```python
from build123d import *

# Parameters (mm, degrees)
SKETCH1_R           = 4.9999999999999964
BOSS_EXTRUDE1_DEPTH = 5
BOSS_EXTRUDE2_DEPTH = 70
BOSS_EXTRUDE3_DEPTH = 70
CUT_EXTRUDE1_DEPTH  = 5
SKETCH6_R           = 20.000000000000004
CUT_EXTRUDE2_DEPTH  = 1
CUT_EXTRUDE3_DEPTH  = 19.000000000000004
BOSS_EXTRUDE4_DEPTH = 1.9999999999999896
FILLET1_R           = 5


with BuildPart() as part:
    # Sketch1 → Boss-Extrude1 (new body)
    with BuildSketch(Plane.XY):
        with BuildLine():
            Line((-7.704615384615421, -40.00000000000001), (32.295384615384584, -40.00000000000001))
            ThreePointArc((32.295384615384584, -40.00000000000001), (72.29538461538459, 0), (32.29538461538458, 39.99999999999999))
            Line((32.29538461538458, 39.99999999999999), (-7.7046153846154315, 39.99999999999999))
            Line((-7.7046153846154315, 39.99999999999999), (-7.704615384615421, -40.00000000000001))
        make_face()
        with Locations((32.295384615384584, 0)):
            Circle(SKETCH1_R, mode=Mode.SUBTRACT)
    boss_extrude1 = extrude(amount=BOSS_EXTRUDE1_DEPTH)

    # Sketch2 → Boss-Extrude2 (add)
    with BuildSketch(Plane.XY.offset(5)):
        Polygon((-7.7046153846154315, 39.99999999999999), (-2.70461538461543, 39.99999999999999), (-2.7046153846154235, -40.00000000000001), (-7.704615384615421, -40.00000000000001), align=None)
    extrude(amount=BOSS_EXTRUDE2_DEPTH)

    # Mirror1: Boss-Extrude1 across plane
    add(boss_extrude1.mirror(Plane.XY.offset(40)))

    # Sketch4 → Boss-Extrude3 (add)
    with BuildSketch(Plane.XY.offset(5)):
        with BuildLine():
            Line((-2.7046153846154266, -40.00000000000001), (-2.7046153846154266, -30.000000000000007))
            Line((-2.7046153846154266, -30.000000000000007), (43.497251593214216, -30.000000000000007))
            Line((43.497251593214216, -30.000000000000007), (58.7528977260305, -30.000000000000007))
            ThreePointArc((58.7528977260305, -30.000000000000007), (46.43752023911554, -37.41657386773942), (32.295384615384584, -40.00000000000001))
            Line((32.295384615384584, -40.00000000000001), (-2.7046153846154266, -40.00000000000001))
        make_face()
    extrude(amount=BOSS_EXTRUDE3_DEPTH)

    # Sketch5 → Cut-Extrude1 (cut)
    with BuildSketch(Plane.ZY.offset(7.704615384615426)):
        with BuildLine():
            ThreePointArc((50.00000000000001, -1.388e-14), (43.82683432365097, 9.238795325112829), (32.92893218813463, 7.071067811865561))
            Line((32.92893218813452, 7.0710678118654755), (47.071067811865476, -7.071067811865483))
            ThreePointArc((47.0710678118656, -7.0710678118653725), (49.2387953251129, -3.826834323650836), (50.00000000000001, -1.633e-14))
        make_face()
        with BuildLine():
            Line((47.071067811865476, -7.071067811865483), (32.92893218813452, 7.0710678118654755))
            ThreePointArc((32.92893218813463, 7.071067811865561), (32.92893218813454, -7.071067811865502), (47.0710678118656, -7.0710678118653725))
        make_face()
    extrude(amount=-CUT_EXTRUDE1_DEPTH, mode=Mode.SUBTRACT)

    # Sketch6 → Cut-Extrude2 (cut)
    with BuildSketch(Plane.ZY.offset(7.704615384615426)):
        with Locations(Location((40.00000000000001, -1.388e-14, 0), (0, 0, 270))):
            Circle(SKETCH6_R)
    extrude(amount=-CUT_EXTRUDE2_DEPTH, mode=Mode.SUBTRACT)

    # Sketch7 → Cut-Extrude3 (cut)
    with BuildSketch(Plane(origin=(0, -30.000000000000007, 0), x_dir=(1, 0, 0), z_dir=(0, 1, 0))):
        Polygon((58.7528977260305, -53.00000000000001), (58.7528977260305, -40.00000000000001), (58.7528977260305, -27.000000000000004), (19.339689979409883, -27.000000000000007), (19.339689979409883, -53.00000000000001), align=None)
    extrude(amount=-CUT_EXTRUDE3_DEPTH, mode=Mode.SUBTRACT)

    # Sketch8 → Boss-Extrude4 (add)
    with BuildSketch(Plane(origin=(0, -30.000000000000007, 0), x_dir=(1, 0, 0), z_dir=(0, 1, 0))):
        Polygon((58.7528977260305, -53.00000000000001), (19.33968997940988, -53.00000000000001), (19.33968997940988, -27.000000000000007), (58.7528977260305, -27.000000000000004), (58.7528977260305, -25.000000000000007), (56.7528977260305, -25.000000000000007), (17.33968997940988, -25.000000000000007), (17.33968997940988, -55.00000000000001), (58.7528977260305, -55.00000000000001), align=None)
    extrude(amount=BOSS_EXTRUDE4_DEPTH)

    # Fillet1
    fillet1_edges = [part.edges().sort_by_distance(p)[0] for p in [
        (-7.704615384615421, -40.00000000000001, 40),
        (28.024141170707534, -30.000000000000007, 5),
        (28.024141170707537, -30.000000000000007, 75),
    ]]
    fillet(fillet1_edges, radius=FILLET1_R)


solid = part.part
```
For this review, take the finished solid that the model builds, in its own axes (mm). A direction names the side the tool comes from. Coordinates: 2 decimals unless noted, no trailing zeros. Order: outer loops, then holes, each group sorted by start corner. A loop starts at its lowest first (then second) coordinate and runs counter-clockwise, first axis right, second up. Notation, with made-up numbers: (-3.5, 69.25) -> (33.5, 69.25) arc R26 cw to (33.5, 83.25) -> close; hole circle Ø5 at (-14, -13.75). An arc over 180 degrees is marked (long way). Answer as CSV lines item,"result".
Q1. Clearance check with flat-ended pins moving along their axes: pin 1 Ø0.6 at (y, z) = (-29.5, 54) entering from +X; pin 2 Ø12 at (x, z) = (55.5, 64.5) entering from +Y; pin 3 Ø6 at (y, z) = (-36, 40) entering from +X; pin 4 Ø18 at (y, z) = (0, 40) entering from +X. State where each tip first meets the part, or that it passes through.
Model answer:
pin 1,"stops at x = 58.75"
pin 2,"stops at y = -29.97"
pin 3,"stops at x = 19.34"
pin 4,"passes through"
Q2. For faces 5 (the face through (34, -34, 27)), 6 (the face through (23, 1, 80)), 7 (the face through (34, 8, 75)), list the 3-axis set-ups (+Z, -Z, +X, -X, +Y, -Y) from which the entire face can be reached by the end or side of a thin tool; tool diameter is ignored.
Model answer:
face 5,"+X, +Y, -Y"
face 6,"+Z, +X, -X, +Y, -Y"
face 7,"+X, +Y"
Q3. We need section B-B (y = 0). State the section outline as (x, z) points, plus the area to 3 significant figures.
Model answer:
outline,"(-7.7, 0) -> (27.3, 0) -> (27.3, 5) -> (-2.7, 5) -> (-2.7, 30) -> (-6.7, 30) -> (-6.7, 20) -> (-7.7, 20) -> close; (-7.7, 60) -> (-6.7, 60) -> (-6.7, 50) -> (-2.7, 50) -> (-2.7, 75) -> (27.3, 75) -> (27.3, 80) -> (-7.7, 80) -> close; (37.3, 0) -> (72.3, 0) -> (72.3, 5) -> (37.3, 5) -> close; (37.3, 75) -> (72.3, 75) -> (72.3, 80) -> (37.3, 80) -> close"
area,"930 mm2"
Q4. Draft analysis for pull direction Y (two halves, no side actions). For faces 1 (the face through (27.3, 0.2, 77.5)), 2 (the face through (-4.733, 5.37, 48.436)), 3 (the face through (31, -29, 7)), 4 (the face through (63.495, -25.031, 75.311)), state which applies: released by +Y, released by -Y, zero draft, split by the parting line, or undercut.
Model answer:
face 1,"undercut"
face 2,"undercut"
face 3,"released by +Y"
face 4,"split by the parting line"
Q5. We need section D-D (y = 29). State the section outline as (x, z) points.
Model answer:
outline,"(-7.7, 0) -> (59.85, 0) -> (59.85, 5) -> (-2.7, 5) -> (-2.7, 75) -> (59.85, 75) -> (59.85, 80) -> (-7.7, 80) -> close"
Q6. We need section C-C (x = 52). State the section outline as (y, z) points.
Model answer:
outline,"(-34.81, 0) -> (34.81, 0) -> (34.81, 5) -> (-25, 5) arc R5 cw to (-30, 10) -> (-30, 25) -> (-28, 25) -> (-28, 27) -> (-34.81, 27) -> close; (-34.81, 53) -> (-28, 53) -> (-28, 55) -> (-30, 55) -> (-30, 70) arc R5 cw to (-25, 75) -> (34.81, 75) -> (34.81, 80) -> (-34.81, 80) -> close"
Q7. We need section A-A (z = 40). State the section outline as (x, y) points, plus the area to 3 significant figures.
Model answer:
outline,"(-7.7, -35) arc R5 ccw to (-2.7, -40) -> (19.34, -40) -> (19.34, -28) -> (17.34, -28) -> (17.34, -30) -> (-2.7, -30) -> (-2.7, -10) -> (-6.7, -10) -> (-6.7, -20) -> (-7.7, -20) -> close; (-7.7, 20) -> (-6.7, 20) -> (-6.7, 10) -> (-2.7, 10) -> (-2.7, 40) -> (-7.7, 40) -> close"
area,"499 mm2"
Q8. Wall thickness on line 1 along Z through (x, y) = (20.5, 0); line 2 along Z through (x, y) = (-7.3, 0); line 3 along Y through (x, z) = (-3, 40): over which ranges is each line inside the solid? List them lowest first. Write a range as [from, to].
Model answer:
line 1,"z = [0, 5], [75, 80]"
line 2,"z = [0, 20], [60, 80]"
line 3,"y = [-39.99, -10], [10, 40]"
